```python
from build123d import *

# Parameters (mm, degrees)
CBORE_FOR_M3_HEX_SOCKET_HEAD_CAP_SCREW1_D           = 3.4
CBORE_FOR_M3_HEX_SOCKET_HEAD_CAP_SCREW1_CBORE_D     = 6.5
CBORE_FOR_M3_HEX_SOCKET_HEAD_CAP_SCREW1_CBORE_DEPTH = 3.4


with BuildPart() as part:
    # Sketch1 → Revolve1 (revolve)
    with BuildSketch(Plane.XY, mode=Mode.PRIVATE) as revolve1_sk:
        Polygon((29, 0), (37, 0), (37, 31), (27, 31), (27, 7), (29, 7), align=None)
    revolve(revolve1_sk.sketch.rotate(Axis((0, 0, 0), (0, 1, 0)), 90), axis=Axis((0, 0, 0), (0, 1, 0)))

    # CBORE for M3 Hex Socket Head Cap Screw1 (through all)
    with Locations(Plane(origin=(0, 0, 0), x_dir=(-1, 0, 0), z_dir=(0, -1, 0))):
        with Locations((28.578838325, -16.5), (0, -33), (-28.578838325, -16.5), (-28.578838325, 16.5), (0, 33), (28.578838325, 16.5)):
            CounterBoreHole(CBORE_FOR_M3_HEX_SOCKET_HEAD_CAP_SCREW1_D / 2, CBORE_FOR_M3_HEX_SOCKET_HEAD_CAP_SCREW1_CBORE_D / 2, CBORE_FOR_M3_HEX_SOCKET_HEAD_CAP_SCREW1_CBORE_DEPTH)


solid = part.part
```
Design review of the part built by this model. Coordinates are the model's own, in mm. A direction names the side the tool comes from. Coordinates: 2 decimals unless noted, no trailing zeros. Order: outer loops, then holes, each group sorted by start corner. A loop starts at its lowest first (then second) coordinate and runs counter-clockwise, first axis right, second up. Notation, with made-up numbers: (39, 48) - (75, 48) arc R32 ccw to (75, 83) - close; hole circle Ø11 at (-30, 43). An arc over 180 degrees is marked (long way). One line per question, with ' | ' between items.
Q1. Consider section D-D, the plane z = -16.5. Give the boundary of the cut face in (x, y).
Answer key:
outline: (-33.12, 0) - (-31.83, 0) - (-31.83, 3.4) - (-30.28, 3.4) - (-30.28, 31) - (-33.12, 31) - close; (-26.88, 3.4) - (-25.33, 3.4) - (-25.33, 0) - (-23.85, 0) - (-23.85, 7) - (-21.37, 7) - (-21.37, 31) - (-26.88, 31) - close; (21.37, 7) - (23.85, 7) - (23.85, 0) - (25.33, 0) - (25.33, 3.4) - (26.88, 3.4) - (26.88, 31) - (21.37, 31) - close; (30.28, 3.4) - (31.83, 3.4) - (31.83, 0) - (33.12, 0) - (33.12, 31) - (30.28, 31) - close
Q2. To check wall thickness, follow line 1 along X through (y, z) = (9.5, -17.5); line 2 along Z through (x, y) = (6, 19.5); line 3 along Z through (x, y) = (-10.5, 25). State the ranges of each line that lie inside material, in increasing order.
Answer key:
line 1: x = -32.6 to -29.95, -27.2 to -20.56, 20.56 to 27.2, 29.95 to 32.6 | line 2: z = -36.51 to -26.32, 26.32 to 36.51 | line 3: z = -35.48 to -24.87, 24.87 to 35.48
Q3. For faces 4 (the cylindrical face through (30.15, 17.39, -15.85)), 5 (the cylindrical face through (25.73, 3.45, -13.38)), list the 3-axis set-ups (+Z, -Z, +X, -X, +Y, -Y) from which the entire face can be reached by the end or side of a thin tool; tool diameter is ignored.
Answer key:
face 4: +Y, -Y | face 5: -Y
Q4. Consider section A-A, the plane y = 27. Give the boundary of the cut face in (x, z).
Answer key:
outline: circle Ø74 at (0, 0); hole circle Ø3.4 at (-28.58, -16.5); hole circle Ø3.4 at (-28.58, 16.5); hole circle Ø54 at (0, 0); hole circle Ø3.4 at (0, -33); hole circle Ø3.4 at (0, 33); hole circle Ø3.4 at (28.58, -16.5); hole circle Ø3.4 at (28.58, 16.5)
Q5. The part is to be moulded in two halves that separate along X. For faces 1 (the cylindrical face through (32.825, 15.717, -17.073)), 2 (the flat face through (-30, 3.4, -15)), 3 (the flat face through (30, 0, -3)), say which applies: +X half, -X half, draft (parallel to the pull), parting line (faces both ways), or undercut.
Answer key:
face 1: parting line | face 2: undercut | face 3: draft
Q6. Consider section C-C, the plane z = -3. Give the boundary of the cut face in (x, y), then the cut area to 3 significant figures.
Answer key:
outline: (-36.88, 0) - (-28.84, 0) - (-28.84, 7) - (-26.83, 7) - (-26.83, 31) - (-36.88, 31) - close; (26.83, 7) - (28.84, 7) - (28.84, 0) - (36.88, 0) - (36.88, 31) - (26.83, 31) - close | area: 595 mm2
Q7. Clearance check with flat-ended pins moving along their axes: pin 1 Ø3 at (x, z) = (-1, -32) entering from -Y; pin 2 Ø2 at (y, z) = (16.5, -16) entering from +X; pin 3 Ø5 at (x, y) = (26.5, 20.5) entering from -Z. State where each tip first meets the part, or that it passes through.
Answer key:
pin 1: stops at y = 3.4 | pin 2: stops at x = 33.82 | pin 3: stops at z = -28.16
Q8. Consider section B-B, the plane x = -15.5. Give the boundary of the cut face in (y, z).
Answer key:
outline: (0, -33.6) - (31, -33.6) - (31, -22.11) - (7, -22.11) - (7, -24.51) - (0, -24.51) - close; (0, 24.51) - (7, 24.51) - (7, 22.11) - (31, 22.11) - (31, 33.6) - (0, 33.6) - close
